Input: part model. Units: mm. Frame: model coordinates. A direction names the side the tool comes from. Round coordinates to 2 decimals unless told otherwise and drop trailing zeros. Order: outer loops, then holes, each group sorted by start corner. A loop starts at its lowest first (then second) coordinate and runs counter-clockwise, first axis right, second up. Notation, with made-up numbers: M 47,-32 L 54,-32 A20 ccw 54,-27 Z; hole C 28,89 d9. An arc over 180 degrees is marked long. One line per question, with ' | ' between items.
```python
from build123d import *

# Parameters (mm, degrees)
F0_W     = 1143
F0_H     = 482.6
F1_DEPTH = 63.5
F2_W     = 203.2
F2_H     = 177.8
F3_DEPTH = 63.5
F4_R     = 12.7
F5_DEPTH = 482.6
F7_DEPTH = 63.5


with BuildPart() as f1:
    # F0 (on Top) → F1 (new body)
    with BuildSketch(Plane.XY):
        with Locations((571.5, 241.3)):
            Rectangle(F0_W, F0_H)
    extrude(amount=F1_DEPTH)

    # F2 (on face) → F3 (cut)
    with BuildSketch(Plane.XY.offset(63.5)):
        with Locations((927.1, 228.6)):
            Rectangle(F2_W, F2_H)
    extrude(amount=-F3_DEPTH, mode=Mode.SUBTRACT)

    # F4 (on face) → F5 (cut, through all)
    with BuildSketch(Plane.XZ):
        with Locations((50.8, 19.05)):
            Circle(F4_R)
    extrude(amount=-F5_DEPTH, mode=Mode.SUBTRACT)

    # F6 (on face) → F7 (join)
    with BuildSketch(Plane.XY.offset(63.5)):
        with BuildLine():
            Line((310.490912, 482.6), (787.4, 482.6))
            Line((787.4, 482.6), (787.4, 596.9))
            Line((787.4, 596.9), (453.776858, 596.9))
            ThreePointArc((453.776858, 596.9), (410.838843, 587.380871), (375.946743, 560.607221))
            Line((375.946743, 560.607221), (310.490912, 482.6))
        make_face()
        with BuildLine():
            Line((787.4, -114.3), (787.4, 0))
            Line((787.4, 0), (310.490912, 0))
            Line((310.490912, 0), (375.946743, -78.007221))
            ThreePointArc((375.946743, -78.007221), (410.838843, -104.780871), (453.776858, -114.3))
            Line((453.776858, -114.3), (787.4, -114.3))
        make_face()
    extrude(amount=-F7_DEPTH)


solid = f1.part
```
Item 1: Section query A-A, the plane x = 50.8. Return loops of the section in (y, z), plus the area to 3 significant figures.
Report:
outline: M 0,0 L 482.6,0 L 482.6,6.35 L 0,6.35 Z; M 0,31.75 L 482.6,31.75 L 482.6,63.5 L 0,63.5 Z | area: 18,400 mm²
Item 2: Section query D-D, the plane y = 547. Return loops of the section in (x, z), plus the area to 3 significant figures.
Report:
outline: M 364.53,0 L 787.4,0 L 787.4,63.5 L 364.53,63.5 Z | area: 26,900 mm²
Item 3: Line query: line 1 along X through (y, z) = (252, 17.5); line 2 along X through (y, z) = (316, 18.5); line 3 along X through (y, z) = (168.5, 44.5). Output: solid intervals per line, ascending. Write a range as from..to.
Report:
line 1: 0..38.19, 63.41..825.5, 1028.7..1143 | line 2: 0..38.11, 63.49..825.5, 1028.7..1143 | line 3: 0..825.5, 1028.7..1143
Item 4: Section query B-B, the plane z = 19.05. Return loops of the section in (x, y), plus the area to 3 significant figures.
Report:
outline: M 0,0 L 38.1,0 L 38.1,482.6 L 0,482.6 Z; M 63.5,0 L 310.49,0 L 375.95,-78.01 A101.6 ccw 453.78,-114.3 L 787.4,-114.3 L 787.4,0 L 1143,0 L 1143,482.6 L 787.4,482.6 L 787.4,596.9 L 453.78,596.9 A101.6 ccw 375.95,560.61 L 310.49,482.6 L 63.5,482.6 Z; hole M 825.5,139.7 L 1028.7,139.7 L 1028.7,317.5 L 825.5,317.5 Z | area: 601,000 mm²
Item 5: Section query C-C, the plane x = 984.5. Return loops of the section in (y, z), plus the area to 3 significant figures.
Report:
outline: M 0,0 L 139.7,0 L 139.7,63.5 L 0,63.5 Z; M 317.5,0 L 482.6,0 L 482.6,63.5 L 317.5,63.5 Z | area: 19,400 mm²
Item 6: First-contact query: pin 1 (19 mm diameter, centred on x = 1038, z = 20.5, fed in from -Y); pin 2 (1.5 mm diameter, centred on y = 506, z = 47, fed in from -X); pin 3 (4 mm diameter, centred on x = 161, z = 34.5, fed in from +Y). Flat tips, straight axial feed; report the tip coordinate or a pass-through.
Report:
pin 1: y = 0 | pin 2: x = 329.5 | pin 3: y = 482.6
Item 7: Access query for faces 5 (the flat face through (825.5, 227, 32)), 6 (the flat face through (787.4, -58, 32)), 7 (the flat face through (618, -114.3, 32)), 8 (the flat face through (153, 0, 31)). Directions: +Z, -Z, +X, -X, +Y, -Y. A direction counts if a zero-diameter tool reaches every point of the face in a straight line with its end or side. Return the directions, or none.
Report:
face 5: +Z, -Z | face 6: +Z, -Z, +X, -Y | face 7: +Z, -Z, +X, -X, -Y | face 8: +Z, -Z, -X, -Y
Item 8: Mould query, pull axis Z, two halves, no side actions, for faces 1 (the flat face through (563, 246, 63.5)), 2 (the cylindrical face through (40.722, 237.922, 11.322)), 3 (the flat face through (787.4, 539, 32)), 4 (the flat face through (563, 246, 0)). Classes: +Z half, -Z half, draft (parallel to the pull), parting line (faces both ways), or undercut.
Report:
face 1: +Z half | face 2: undercut | face 3: draft | face 4: -Z half
